from build123d import *

# Parameters (mm, degrees)
PAD001_DEPTH    = 8
SKETCH009_W     = 6
SKETCH009_H     = 10
PAD004_DEPTH    = 2
POCKET005_DEPTH = 11.051
CHAMFER_SIZE    = 0.5


with BuildPart() as part:
    # Sketch003 → Pad001 (new body)
    with BuildSketch(Plane.YZ):
        Polygon((-3.05, 2.5), (-8.05, -2.5), (8.05, -2.5), (3.05, 2.5), (3.05, -0.55), (-3.05, -0.55), align=None)
    extrude(amount=PAD001_DEPTH)

    # Sketch009 (on Face2 of Pad001) → Pad004 (join)
    with BuildSketch(Plane.YX.offset(2.5)):
        with Locations((0, 4)):
            Rectangle(SKETCH009_W, SKETCH009_H)
    extrude(amount=-PAD004_DEPTH)

    # Sketch010 (on Face8 of Pad004) → Pocket005 (cut, through all)
    with BuildSketch(Plane(origin=(0, -3, 0), x_dir=(0, 0, -1), z_dir=(0, -1, 0))):
        Polygon((2.5, 9), (0.5, 9), (0.5, 8), align=None)
        Polygon((2.5, -1), (0.5, -1), (0.5, 0), align=None)
    extrude(amount=-POCKET005_DEPTH, mode=Mode.SUBTRACT)

    # Chamfer
    chamfer_edges = [part.edges().sort_by_distance(p)[0] for p in [
        (4, -3.05, 2.5),
        (4, 3.05, 2.5),
        (4, -8.05, -2.5),
        (4, 8.05, -2.5),
    ]]
    chamfer(chamfer_edges, length=CHAMFER_SIZE)


with BuildPart() as part_1:
    # Body001 placement: moved
    add(part.part.moved(Location((8.5, -3, -20.5))))


solid = part_1.part
Source: CAD feature listing. Evaluate the final solid. Frame: model axes, mm. A direction names the side the tool comes from. Round coordinates to 2 decimals unless told otherwise and drop trailing zeros. Write each loop counter-clockwise with the first axis right and the second up, starting at its lowest first coordinate (ties: lowest second). Pieces come first, ordered by that corner, then holes. Notation, with made-up numbers: M 64.25,0 L 81.25,0 A29 cw 81.25,33 Z; hole C -24,-25 d7. An arc over 180 degrees is marked long. One line per item, written item: value. Start each with the question number.
Item 1: Mould query, pull axis Y, two halves, no side actions, for faces 1 (the flat face through (12.44, -8.52, -20.47)), 2 (the flat face through (16.5, 2, -21)), 3 (the flat face through (12, 0.05, -20)). Classes: pulls with the +Y half, pulls with the -Y half, needs draft (parallel to the pull), parting line crosses it, or undercut.
Item 2: Set-up query: faces 4 (the flat face through (13, -3, -21)), 5 (the flat face through (8.5, -8, -21)), 6 (the flat face through (8.5, 2, -21)), 7 (the flat face through (16.5, -8, -21)). Return all of +Z, -Z, +X, -X, +Y, -Y with unobstructed straight access to the full face (end or side cutting, diameter ignored); none if empty.
Item 3: Pin query (flat end, axial travel): pin 1 (0.6 mm diameter, centred on x = 11, z = -22, fed in from -Y); pin 2 (1 mm diameter, centred on y = -7, z = -21, fed in from -X); pin 3 (2 mm diameter, centred on x = 14, z = -20, fed in from -Y). Return the tip coordinate at first contact, or that it passes through.
Item 4: Section query D-D (y = -1.75). Return the cut outline in (x, z).
Item 5: Section query A-A (z = -18.75). Return the cut outline in (x, y).
Item 6: Ray query, L1, parallel to Y at x = 16, z = -20.65; L2, parallel to Z at x = 13.5, y = -4.25; L3, parallel to Y at x = 9.5, z = -20.05. Return the intervals inside material, ascending. Write a range as from..to.
Item 7: Section query C-C (x = 11.75). Return the cut outline in (y, z).
Item 8: Section query B-B (z = -22.1). Return the cut outline in (x, y).
Result set:
1. face 1: pulls with the -Y half
1. face 2: needs draft
1. face 3: undercut
2. face 4: +Z, +X, -X
2. face 5: +Z, -Z, -X, -Y
2. face 6: +Z, -Z, -X, +Y
2. face 7: +Z, -Z, +X, -Y
3. pin 1: stops at y = -10.35
3. pin 2: stops at x = 8.5
3. pin 3: stops at y = -9.05
4. outline: M 7.5,-23 L 17.5,-23 L 16.5,-21 L 8.5,-21 Z
5. outline: M 8.5,-6.8 L 16.5,-6.8 L 16.5,-6.05 L 8.5,-6.05 Z; M 8.5,0.05 L 16.5,0.05 L 16.5,0.8 L 8.5,0.8 Z
6. L1: y = -8.7..-6.05, 0.05..2.7
6. L2: z = -23..-21
6. L3: y = -8.1..-6.05, 0.05..2.1
7. outline: M -10.7,-22.65 L -10.55,-23 L 4.55,-23 L 4.7,-22.65 L 0.4,-18.35 L 0.05,-18.5 L 0.05,-21.05 L 0,-21.05 L 0,-21 L -6,-21 L -6,-21.05 L -6.05,-21.05 L -6.05,-18.5 L -6.4,-18.35 Z
8. outline: M 7.95,-6 L 8.5,-6 L 8.5,-10.15 L 16.5,-10.15 L 16.5,-6 L 17.05,-6 L 17.05,0 L 16.5,0 L 16.5,4.15 L 8.5,4.15 L 8.5,0 L 7.95,0 Z
